The figure shows three views and two pictorial views of one solid part (mm, origin at its lowest corner). Answer the questions. Give positions to 0.01 mm unless a question says otherwise; leave off trailing zeros. Order: outer loops, then holes, each group sorted by start corner. A loop starts at its lowest first (then second) coordinate and runs counter-clockwise, first axis right, second up. Notation, with made-up numbers: M 58,79.5 L 76,79.5 A19 ccw 76,86.5 Z; hole C 7.25,41.25 d5. An arc over 180 degrees is marked long. One line per item, written item: value.
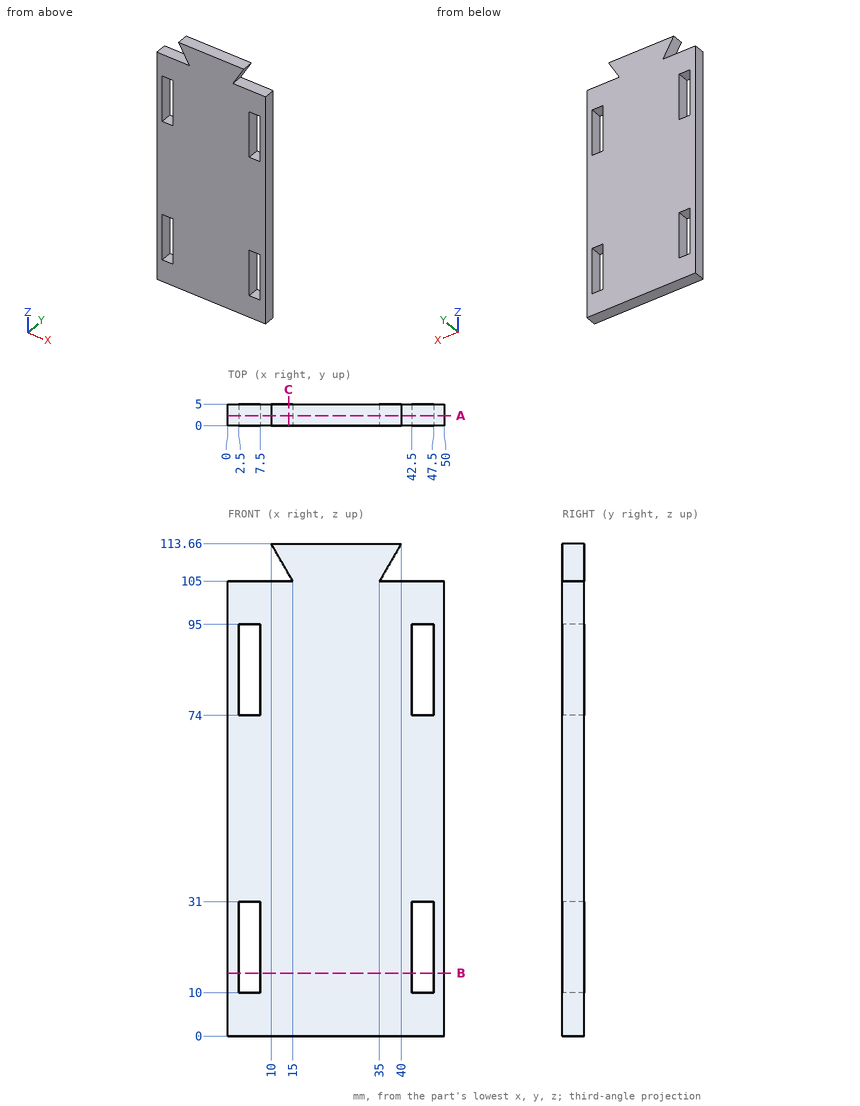
1) This flat-tipped pin is pushed along its axis until it touches: pin 1 Ø1.5 at (x, y) = (5, 1.5) entering from +Z. Where does it stop, or does it pass through?
Reported:
pin 1: stops at z = 105
2) Find section B-B, the plane z = 14.5. Write down the section's boundary in (x, y).
Reported:
outline: M 0,0 L 2.5,0 L 2.5,5 L 0,5 Z; M 7.5,0 L 42.5,0 L 42.5,5 L 7.5,5 Z; M 47.5,0 L 50,0 L 50,5 L 47.5,5 Z
3) Consider probe 1 along X at (y, z) = (3.5, 15.5); probe 2 along Z at (x, y) = (3.5, 0.4); probe 3 along Z at (x, y) = (48, 2.2). Determine where each line is inside the solid, lowest interval first.
Reported:
probe 1: x = 0 to 2.5, 7.5 to 42.5, 47.5 to 50
probe 2: z = 0 to 10, 31 to 74, 95 to 105
probe 3: z = 0 to 105
4) Find section A-A, the plane y = 2.3. Write down the section's boundary in (x, z), plus the area to 3 significant figures.
Reported:
outline: M 0,0 L 50,0 L 50,105 L 35,105 L 40,113.66 L 10,113.66 L 15,105 L 0,105 Z; hole M 2.5,10 L 7.5,10 L 7.5,31 L 2.5,31 Z; hole M 2.5,74 L 7.5,74 L 7.5,95 L 2.5,95 Z; hole M 42.5,10 L 47.5,10 L 47.5,31 L 42.5,31 Z; hole M 42.5,74 L 47.5,74 L 47.5,95 L 42.5,95 Z
area: 5,050 mm^2
5) Find section C-C, the plane x = 14. Write down the section's boundary in (y, z).
Reported:
outline: M 0,0 L 5,0 L 5,105 L 0,105 Z; M 0,106.73 L 5,106.73 L 5,113.66 L 0,113.66 Z
